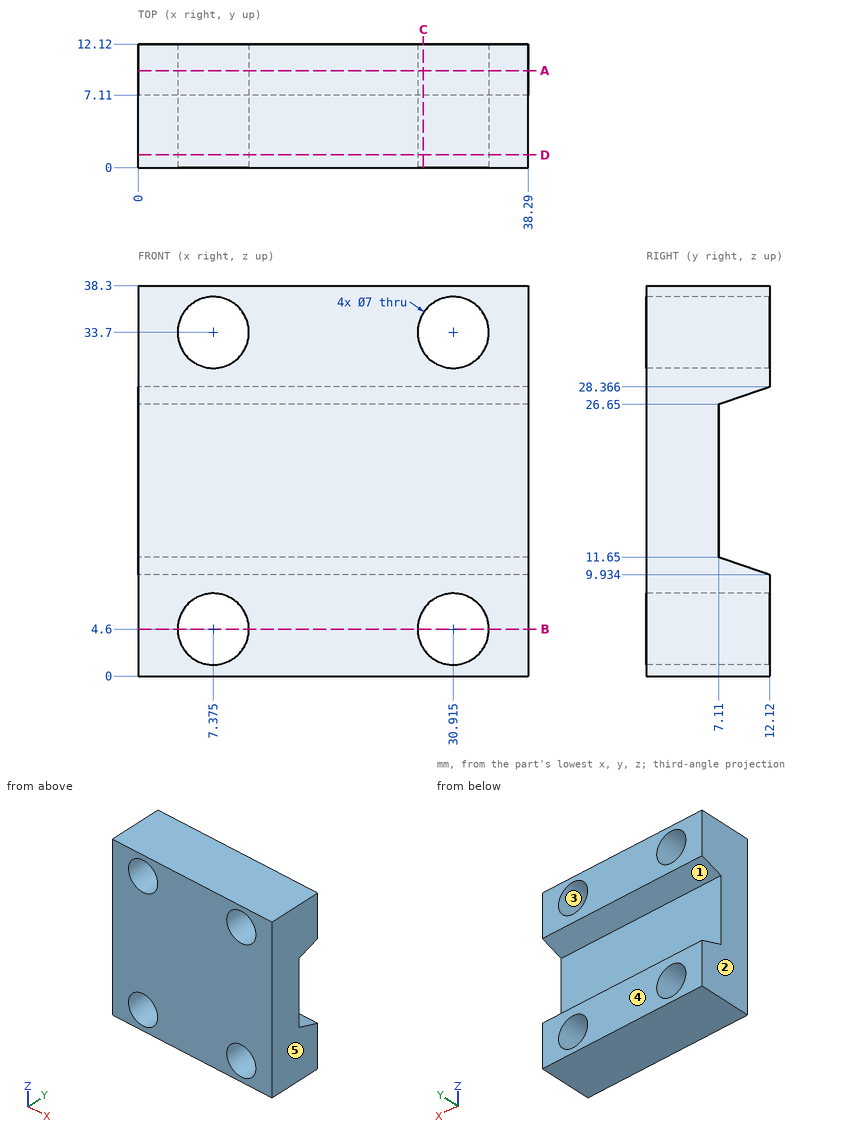
Design review of the part shown in the three views and the two pictorial views. Dimensions are in mm from the part's minimum x, y and z. A direction names the side the tool comes from. Round coordinates to 2 decimals unless told otherwise and drop trailing zeros. Write each loop counter-clockwise with the first axis right and the second up, starting at its lowest first coordinate (ties: lowest second). Pieces come first, ordered by that corner, then holes.
Item 1: We need section C-C on x = 28. Write out the cut boundary in (y, z).
Item 2: We need section D-D on y = 1.25. Write out the cut boundary in (x, z) (1 decimal), and give its area (3 significant figures).
Item 3: For the marked faces 1 and 2, list the 3-axis set-ups (+Z, -Z, +X, -X, +Y, -Y) from which the entire face can be reached by the end or side of a thin tool; tool diameter is ignored.
Item 4: For probe 1 along Z at (x, y) = (31, 4); probe 2 along X at (y, z) = (8, 33.7) (1 decimal); probe 3 along Z at (x, y) = (29.5, 4.25), list the stretches that pass through material, from the lowest coordinate up.
Item 5: We need section A-A on y = 9.5. Write out the cut boundary in (x, z) (1 decimal).
Item 6: We need section B-B on z = 4.6. Write out the cut boundary in (x, y) (1 decimal), and give its area (3 significant figures).
Item 7: The part is to be moulded in two halves that separate along X. For the marked faces 3, 4 and 5, say which applies: +X half, -X half, draft (parallel to the pull), parting line (faces both ways), or undercut.
Returned:
1. outline: (0, 0) - (12.12, 0) - (12.12, 2.66) - (0, 2.66) - close; (0, 6.54) - (12.12, 6.54) - (12.12, 9.93) - (7.11, 11.65) - (7.11, 26.65) - (12.12, 28.37) - (12.12, 31.76) - (0, 31.76) - close; (0, 35.64) - (12.12, 35.64) - (12.12, 38.3) - (0, 38.3) - close
2. outline: (0, 0) - (38.3, 0) - (38.3, 38.3) - (0, 38.3) - close; hole circle Ø7 at (7.4, 4.6); hole circle Ø7 at (7.4, 33.7); hole circle Ø7 at (30.9, 4.6); hole circle Ø7 at (30.9, 33.7)
2. area: 1,310 mm2
3. face 1: +X, -X, +Y
3. face 2: +Z, -Z, -X, +Y, -Y
4. probe 1: z = 0 to 1.1, 8.1 to 30.2, 37.2 to 38.3
4. probe 2: x = 0 to 3.9, 10.9 to 27.4, 34.4 to 38.3
4. probe 3: z = 0 to 1.4, 7.8 to 30.5, 36.9 to 38.3
5. outline: (0, 0) - (38.3, 0) - (38.3, 10.8) - (0, 10.8) - close; (0, 27.5) - (38.3, 27.5) - (38.3, 38.3) - (0, 38.3) - close; hole circle Ø7 at (7.4, 4.6); hole circle Ø7 at (7.4, 33.7); hole circle Ø7 at (30.9, 4.6); hole circle Ø7 at (30.9, 33.7)
6. outline: (0, 0) - (3.9, 0) - (3.9, 12.1) - (0, 12.1) - close; (10.9, 0) - (27.4, 0) - (27.4, 12.1) - (10.9, 12.1) - close; (34.4, 0) - (38.3, 0) - (38.3, 12.1) - (34.4, 12.1) - close
6. area: 294 mm2
7. face 3: undercut
7. face 4: draft
7. face 5: +X half
